from build123d import *

# Parameters (mm, degrees)
F1_DEPTH = 6.35


with BuildPart() as f1:
    # F0 (on Front) → F1 (new body)
    with BuildSketch(Plane.XZ):
        with BuildLine():
            Line((-13.917371, -25.4), (-13.917371, -19.05))
            ThreePointArc((-13.917371, -19.05), (-10.742371, -15.875), (-7.567371, -19.05))
            Line((-7.567371, -19.05), (7.567371, -19.05))
            ThreePointArc((7.567371, -19.05), (10.742371, -15.875), (13.917371, -19.05))
            Line((13.917371, -19.05), (13.917371, -25.4))
            Line((13.917371, -25.4), (32.227114, -25.4))
            Line((32.227114, -25.4), (32.227114, -9.4996))
            Line((32.227114, -9.4996), (24.659743, -9.4996))
            ThreePointArc((24.659743, -9.4996), (22.414679, -8.569664), (21.484743, -6.3246))
            Line((21.484743, -6.3246), (21.484743, 6.3246))
            ThreePointArc((21.484743, 6.3246), (22.414679, 8.569664), (24.659743, 9.4996))
            Line((24.659743, 9.4996), (32.227114, 9.4996))
            Line((32.227114, 9.4996), (32.227114, 25.4))
            Line((32.227114, 25.4), (13.917371, 25.4))
            Line((13.917371, 25.4), (13.917371, 19.05))
            ThreePointArc((13.917371, 19.05), (10.742371, 15.875), (7.567371, 19.05))
            Line((7.567371, 19.05), (-7.567371, 19.05))
            ThreePointArc((-7.567371, 19.05), (-10.742371, 15.875), (-13.917371, 19.05))
            Line((-13.917371, 19.05), (-13.917371, 25.4))
            Line((-13.917371, 25.4), (-32.227113, 25.4))
            Line((-32.227113, 25.4), (-32.227113, 9.4996))
            Line((-32.227113, 9.4996), (-24.659742, 9.4996))
            ThreePointArc((-24.659742, 9.4996), (-22.414678, 8.569664), (-21.484742, 6.3246))
            Line((-21.484742, 6.3246), (-21.484742, -6.3246))
            ThreePointArc((-21.484742, -6.3246), (-22.414678, -8.569664), (-24.659742, -9.4996))
            Line((-24.659742, -9.4996), (-32.227113, -9.4996))
            Line((-32.227113, -9.4996), (-32.227113, -25.4))
            Line((-32.227113, -25.4), (-13.917371, -25.4))
        make_face()
        with BuildLine():
            Line((-7.567371, 9.4996), (7.567371, 9.4996))
            ThreePointArc((7.567371, 9.4996), (9.812435, 8.569664), (10.742371, 6.3246))
            Line((10.742371, 6.3246), (10.742371, -6.3246))
            ThreePointArc((10.742371, -6.3246), (9.812435, -8.569664), (7.567371, -9.4996))
            Line((7.567371, -9.4996), (-7.567371, -9.4996))
            ThreePointArc((-7.567371, -9.4996), (-9.812435, -8.569664), (-10.742371, -6.3246))
            Line((-10.742371, -6.3246), (-10.742371, 6.3246))
            ThreePointArc((-10.742371, 6.3246), (-9.812435, 8.569664), (-7.567371, 9.4996))
        make_face(mode=Mode.SUBTRACT)
    extrude(amount=F1_DEPTH)


solid = f1.part
The listing builds one solid part. Answer for the finished solid, in the listing's coordinates (mm). A direction names the side the tool comes from. Coordinates: 2 decimals unless noted, no trailing zeros. Loops run counter-clockwise (first coordinate to the right, second up) from the corner with the lowest first, then second, coordinate; pieces in that order, holes last. Notation, with made-up numbers: (7.25, -4.75) -> (38.25, -4.75) arc R16 cw to (38.25, 1.25) -> close; hole circle Ø9 at (38.5, -22.5). An arc over 180 degrees is marked (long way). Write item = value, one per line. Start each with the question number.
1) Given pin 1 Ø1 at (x, y) = (-10, -3.5) entering from +Z; pin 2 Ø1.9 at (x, y) = (-3, -3.5) entering from -Z; pin 3 Ø1.5 at (y, z) = (-3.5, 8) entering from +X, each flat-ended and moving along its own axis, determine where each tip first touches the part or whether it passes through.
2) A tool of negligible diameter and unlimited length cuts with its end or side. For faces 5 (the face through (22.439, -3.131, -8.594)), 6 (the face through (-10.742, -3, 0)), 7 (the face through (0, -3, 19.05)), 8 (the face through (-13.917, -3, -22)), 9 (the face through (-22.39, -3.131, -8.545)), from which of +Z, -Z, +X, -X, +Y, -Y can it reach the whole face along a straight path? Write none if from no direction.
3) Straight lines are drawn through the part: line 1 (Z direction, x = 3, y = -3.75); line 2 (X direction, y = -3.5, z = -22); line 3 (Z direction, x = -25.5, y = -5). For each, find the intervals that lie inside material, in ascending order. Write a range as from..to.
4) The mould has two halves that part along Z. Classify faces 1 (the face through (-13.917, -3, 22)), 2 (the face through (23, -3, 25.4)), 3 (the face through (0, -3, -19.05)), 4 (the face through (28, -3, -9.5)): released by +Z, released by -Z, zero draft, split by the parting line, or undercut.
5) A cutting plane is placed at A-A (x = 0). Give the vertices of the cut face in (y, z).
6) A cutting plane is placed at B-B (z = 21). Give the vertices of the cut face in (x, y), then the cut area to 3 significant figures.
Responses:
q1.pin_1 = 16.13
q1.pin_2 = -19.05
q1.pin_3 = 22.61
q2.face_5 = +X, +Y, -Y
q2.face_6 = +Y, -Y
q2.face_7 = +Z, +Y, -Y
q2.face_8 = -Z, +Y, -Y
q2.face_9 = -X, +Y, -Y
q3.line_1 = -19.05..-9.5, 9.5..19.05
q3.line_2 = -32.23..-13.92, 13.92..32.23
q3.line_3 = -25.4..-9.5, 9.5..25.4
q4.face_1 = zero draft
q4.face_2 = released by +Z
q4.face_3 = released by -Z
q4.face_4 = undercut
q5.outline = (-6.35, -19.05) -> (0, -19.05) -> (0, -9.5) -> (-6.35, -9.5) -> close; (-6.35, 9.5) -> (0, 9.5) -> (0, 19.05) -> (-6.35, 19.05) -> close
q6.outline = (-32.23, -6.35) -> (-13.92, -6.35) -> (-13.92, 0) -> (-32.23, 0) -> close; (13.92, -6.35) -> (32.23, -6.35) -> (32.23, 0) -> (13.92, 0) -> close
q6.area = 233 mm²
